Geometry: see drawing. Coordinates: mm, zero at the bounding-box minimum. A direction names the side the tool comes from. Round coordinates to 2 decimals unless told otherwise and drop trailing zeros. Order: outer loops, then holes, each group sorted by start corner. A loop starts at its lowest first (then second) coordinate and runs counter-clockwise, first axis right, second up. Notation, with made-up numbers: (61, -8.75) -> (97, -8.75) arc R26 ccw to (97, 17.25) -> close; hole circle Ø6 at (-13, -16.5). An arc over 180 degrees is marked (long way). Put each result on its own line as item: value.
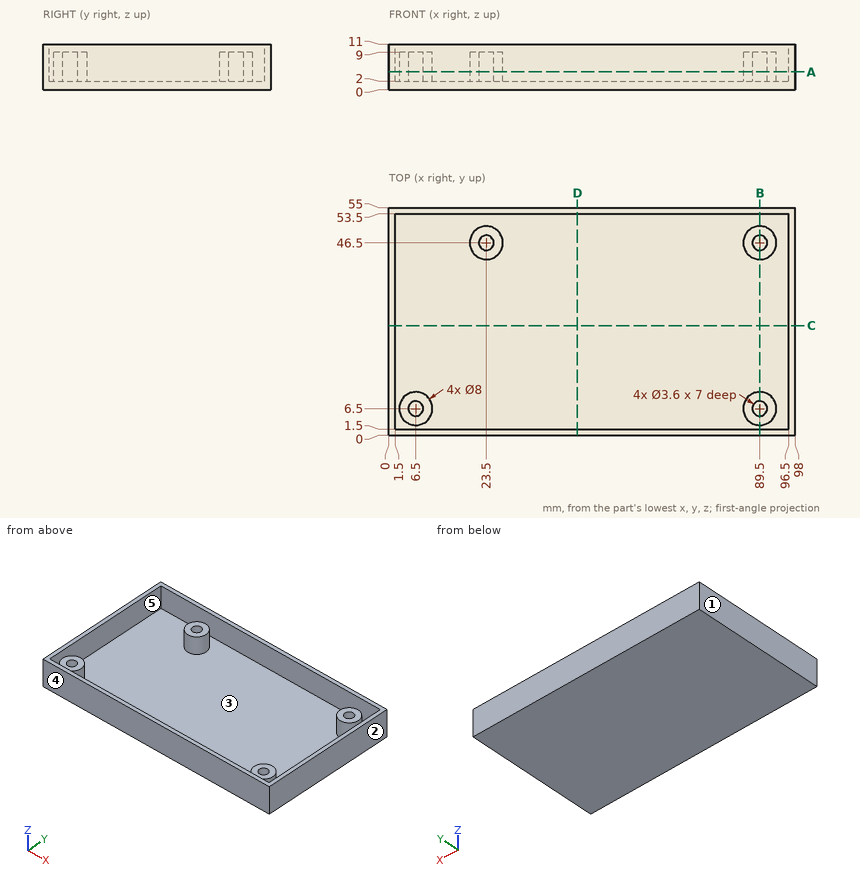
1. Cut plane B-B on x = 89.5. Return loops of the section in (y, z), and give its area (3 significant figures).
Ans:
outline: (0, 0) -> (55, 0) -> (55, 11) -> (53.5, 11) -> (53.5, 2) -> (50.5, 2) -> (50.5, 9) -> (48.3, 9) -> (48.3, 2) -> (44.7, 2) -> (44.7, 9) -> (42.5, 9) -> (42.5, 2) -> (10.5, 2) -> (10.5, 9) -> (8.3, 9) -> (8.3, 2) -> (4.7, 2) -> (4.7, 9) -> (2.5, 9) -> (2.5, 2) -> (1.5, 2) -> (1.5, 11) -> (0, 11) -> close
area: 199 mm²
2. Draft query along X for the marked faces 1, 2 and 3. Return one class per face: +X half, -X half, draft (parallel to the pull), parting line (faces both ways), or undercut.
Ans:
face 1: -X half
face 2: +X half
face 3: undercut
3. Cut plane A-A on z = 4.25. State how many separate pieces and enclosed holes the cut face has, and give its area (3 significant figures).
Ans:
separate pieces: 5
enclosed holes: 5
area: 610 mm²
4. Cut plane C-C on y = 26.5. Return loops of the section in (x, z), and give its area (3 significant figures).
Ans:
outline: (0, 0) -> (98, 0) -> (98, 11) -> (96.5, 11) -> (96.5, 2) -> (1.5, 2) -> (1.5, 11) -> (0, 11) -> close
area: 223 mm²
5. Set-up query: the marked faces 4 and 5. Return all of +Z, -Z, +X, -X, +Y, -Y with unobstructed straight access to the full face (end or side cutting, diameter ignored); none if empty.
Ans:
face 4: +Z, -Z, +X, -X, -Y
face 5: +Z
6. Contact query for flat-ended pins moving along their axis: P1, Ø1.1, axis at x = 24.5, y = 47.5, coming from the +Z side; P2, Ø1.5, axis at x = 65, y = 23.5, coming from the +Z side. Output: stop coordinate, or through.
Ans:
P1: z = 9
P2: z = 2
7. Material intervals for probe 1 along Y at (x, z) = (23.5, 4.75); probe 2 along Y at (x, z) = (6.5, 6.75); probe 3 along Y at (x, z) = (89.5, 6), sorted ascending.
Ans:
probe 1: 0 to 1.5, 42.5 to 44.7, 48.3 to 50.5, 53.5 to 55
probe 2: 0 to 1.5, 2.5 to 4.7, 8.3 to 10.5, 53.5 to 55
probe 3: 0 to 1.5, 2.5 to 4.7, 8.3 to 10.5, 42.5 to 44.7, 48.3 to 50.5, 53.5 to 55
8. Cut plane D-D on x = 45.5. Return loops of the section in (y, z).
Ans:
outline: (0, 0) -> (55, 0) -> (55, 11) -> (53.5, 11) -> (53.5, 2) -> (1.5, 2) -> (1.5, 11) -> (0, 11) -> close
